Verification items for this drawing (mm, ordinates from the low corner). Coordinates: 2 decimals unless noted, no trailing zeros. Loops run counter-clockwise (first coordinate to the right, second up) from the corner with the lowest first, then second, coordinate; pieces in that order, holes last. Notation, with made-up numbers: M 78,68.5 L 93,68.5 A32 cw 93,97.5 Z; hole C 9,-40 d4. An arc over 180 degrees is marked long. Return JSON: item names as keys, results as strings.
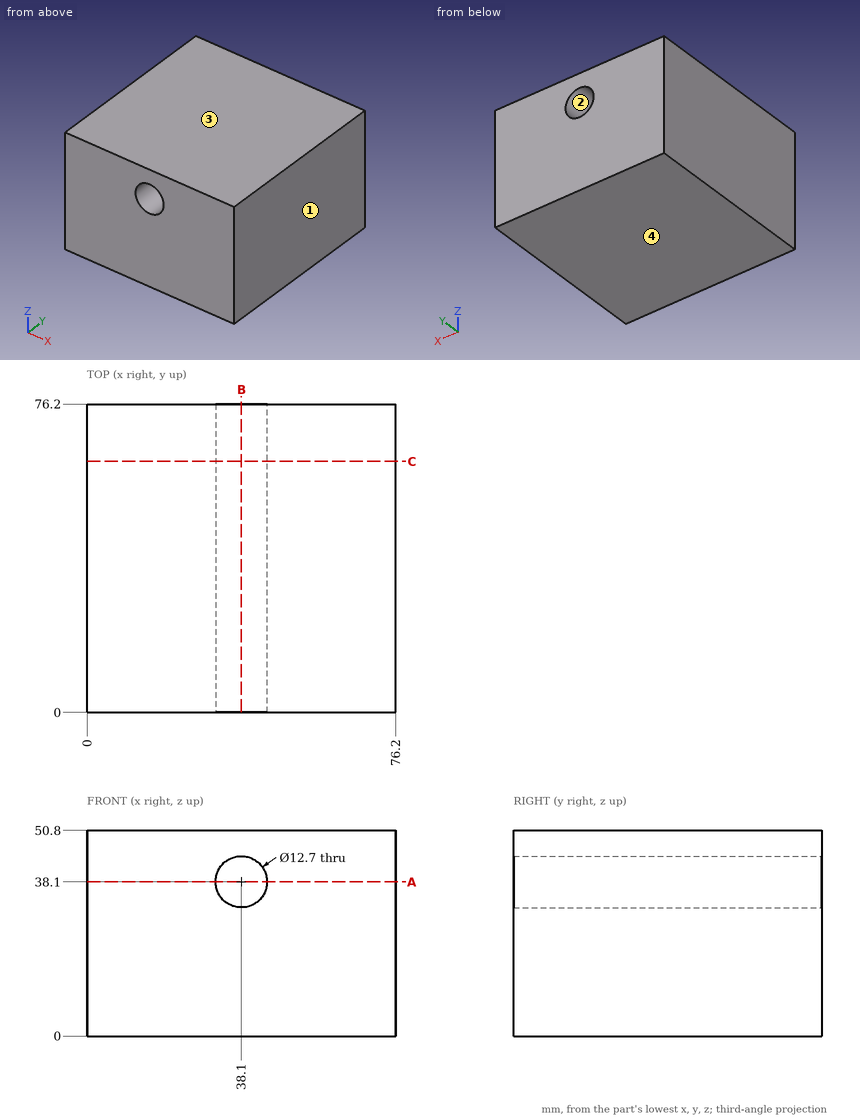
1) Section check C-C on y = 62. Record the cut outline in (x, z).
Answers:
{"outline": "M 0,0 L 76.2,0 L 76.2,50.8 L 0,50.8 Z; hole C 38.1,38.1 d12.7"}
2) Scan lines: line 1 along Z through (x, y) = (38, 18); line 2 along X through (y, z) = (25, 38); line 3 along X through (y, z) = (49, 35.5). Record each from-to range of solid material in increasing order. Write a range as [from, to].
Answers:
{"line 1": "[0, 31.75], [44.45, 50.8]", "line 2": "[0, 31.75], [44.45, 76.2]", "line 3": "[0, 32.31], [43.89, 76.2]"}
3) Draft check along Z on the marked faces 1, 2, 3 and 4. Enter one of: +Z half, -Z half, draft (parallel to the pull), parting line (faces both ways), or undercut.
Answers:
{"face 1": "draft", "face 2": "undercut", "face 3": "+Z half", "face 4": "-Z half"}
4) Section check B-B on x = 38.1. Record the cut outline in (y, z), then the cut area to 3 significant figures.
Answers:
{"outline": "M 0,0 L 76.2,0 L 76.2,31.75 L 0,31.75 Z; M 0,44.45 L 76.2,44.45 L 76.2,50.8 L 0,50.8 Z", "area": "2,900 mm²"}
5) Section check A-A on z = 38.1. Record the cut outline in (x, y).
Answers:
{"outline": "M 0,0 L 31.75,0 L 31.75,76.2 L 0,76.2 Z; M 44.45,0 L 76.2,0 L 76.2,76.2 L 44.45,76.2 Z"}
